The model under review builds one solid part; all positions refer to its coordinate system, in mm. A direction names the side the tool comes from. Coordinates: 2 decimals unless noted, no trailing zeros. Write each loop counter-clockwise with the first axis right and the second up, starting at its lowest first coordinate (ties: lowest second). Pieces come first, ordered by that corner, then holes. Notation, with made-up numbers: (47, 50.5) - (88, 50.5) arc R23 ccw to (88, 59.5) - close; hole circle Ø6 at (-22.75, 45). An arc over 180 degrees is marked (long way). Put each result on its own line as item: value.
from build123d import *

# Parameters (mm, degrees)
RESSALTO_EXTRUS_O1_DEPTH = 1.4
ESBO_O2_R                = 3.45
RESSALTO_EXTRUS_O2_DEPTH = 2.4
FURO4_D                  = 1.2
PADR_O_LINEAR1_COUNT     = 6
PADR_O_LINEAR1_PITCH     = 2
PADR_OCIRCULAR2_COUNT    = 2
PADR_OCIRCULAR2_COPY_1_D = 1.2
PADR_OCIRCULAR2_COPY_2_D = 1.2
PADR_OCIRCULAR2_COPY_3_D = 1.2
PADR_OCIRCULAR2_COPY_4_D = 1.2
PADR_OCIRCULAR2_COPY_5_D = 1.2
FURO1_D                  = 4.95
FURO1_DEPTH              = 2
FURO2_D                  = 4.6
FURO2_DEPTH              = 1
FURO3_D                  = 2.1


with BuildPart() as part:
    # Esboço1 → Ressalto-extrusão1 (new body)
    with BuildSketch(Plane(origin=(0, 0, 0), x_dir=(1, 0, 0), z_dir=(0, 1, 0))):
        with BuildLine():
            Line((-14.159121967, 1.99702088), (-2.209072203, 2.65))
            ThreePointArc((-2.209072203, 2.65), (3.45, 0), (-2.209072203, -2.65))
            Line((-2.209072203, -2.65), (-14.159121967, -1.99702088))
            ThreePointArc((-14.159121967, -1.99702088), (-16.05, 0), (-14.159121967, 1.99702088))
        make_face()
    ressalto_extrus_o1 = extrude(amount=-RESSALTO_EXTRUS_O1_DEPTH)

    # Esboço2 → Ressalto-extrusão2 (add)
    with BuildSketch(Plane.XZ.offset(1.4)):
        with Locations(Location((0, 0, 0), (0, 0, 90))):
            Circle(ESBO_O2_R)
    extrude(amount=RESSALTO_EXTRUS_O2_DEPTH)

    # Furo4 (through all)
    with Locations(Plane(origin=(0, 0, 0), x_dir=(1, 0, 0), z_dir=(0, 1, 0))):
        with Locations((-14.45, 0)):
            furo4 = Hole(FURO4_D / 2)

    # Padrão linear1: Furo4 ×6
    with Locations(*[(i * PADR_O_LINEAR1_PITCH, 0, 0) for i in range(1, PADR_O_LINEAR1_COUNT)]):
        add(furo4, mode=Mode.SUBTRACT)

    # PadrãoCircular2: Ressalto-extrusão1, Furo4 ×2 about axis
    padr_ocircular2_axis = Axis((0, 0, 0), (0, 1, 0))
    add([ressalto_extrus_o1.rotate(padr_ocircular2_axis, i * 360 / PADR_OCIRCULAR2_COUNT) for i in range(1, PADR_OCIRCULAR2_COUNT)])
    add([furo4.rotate(padr_ocircular2_axis, i * 360 / PADR_OCIRCULAR2_COUNT) for i in range(1, PADR_OCIRCULAR2_COUNT)], mode=Mode.SUBTRACT)

    # PadrãoCircular2 copy 1 (through all)
    with Locations(Plane(origin=(-2, 0, 0), x_dir=(-1, 0, 0), z_dir=(0, 1, 0))):
        with Locations((-14.45, 0)):
            Hole(PADR_OCIRCULAR2_COPY_1_D / 2)

    # PadrãoCircular2 copy 2 (through all)
    with Locations(Plane(origin=(-4, 0, 0), x_dir=(-1, 0, 0), z_dir=(0, 1, 0))):
        with Locations((-14.45, 0)):
            Hole(PADR_OCIRCULAR2_COPY_2_D / 2)

    # PadrãoCircular2 copy 3 (through all)
    with Locations(Plane(origin=(-6, 0, 0), x_dir=(-1, 0, 0), z_dir=(0, 1, 0))):
        with Locations((-14.45, 0)):
            Hole(PADR_OCIRCULAR2_COPY_3_D / 2)

    # PadrãoCircular2 copy 4 (through all)
    with Locations(Plane(origin=(-8, 0, 0), x_dir=(-1, 0, 0), z_dir=(0, 1, 0))):
        with Locations((-14.45, 0)):
            Hole(PADR_OCIRCULAR2_COPY_4_D / 2)

    # PadrãoCircular2 copy 5 (through all)
    with Locations(Plane(origin=(-10, 0, 0), x_dir=(-1, 0, 0), z_dir=(0, 1, 0))):
        with Locations((-14.45, 0)):
            Hole(PADR_OCIRCULAR2_COPY_5_D / 2)

    # Furo1
    with Locations(Plane(origin=(0, -3.8, 0), x_dir=(-1, 0, 0), z_dir=(0, -1, 0))):
        with Locations((0, 0)):
            Hole(FURO1_D / 2, depth=FURO1_DEPTH)

    # Furo2
    with Locations(Plane(origin=(0, 0, 0), x_dir=(1, 0, 0), z_dir=(0, 1, 0))):
        with Locations((0, 0)):
            Hole(FURO2_D / 2, depth=FURO2_DEPTH)

    # Furo3 (through all)
    with Locations(Plane(origin=(0, 0, 0), x_dir=(1, 0, 0), z_dir=(0, 1, 0))):
        with Locations((0, 0)):
            Hole(FURO3_D / 2)


solid = part.part
1. The part is to be moulded in two halves that separate along X. For faces 4 (the cylindrical face through (13.004, -0.71, -0.23)), 5 (the flat face through (0, 0, 3)), 6 (the flat face through (-8.1, -0.69, 2.33)), 7 (the cylindrical face through (15.004, -0.71, -0.23)), say which applies: +X half, -X half, draft (parallel to the pull), parting line (faces both ways), or undercut.
Determined:
face 4: undercut
face 5: draft
face 6: -X half
face 7: undercut
2. Machinability: for faces 1 (the cylindrical face through (16.05, -0.69, -0.04)), 2 (the cylindrical face through (2.36, -2.79, -0.74)), 3 (the flat face through (-1, -1, -1)), which of the approach directions +Z, -Z, +X, -X, +Y, -Y give a long, thin tool a straight path to every point of the face, cutting with its end or side? Answer none if there is none.
Determined:
face 1: +X, +Y, -Y
face 2: -Y
face 3: +Y
3. Consider section A-A on x = -6.45. State the section outline as (y, z) points, plus the area to 3 significant figures.
Determined:
outline: (-1.4, -2.42) - (0, -2.42) - (0, -0.6) - (-1.4, -0.6) - close; (-1.4, 0.6) - (0, 0.6) - (0, 2.42) - (-1.4, 2.42) - close
area: 5.09 mm^2
4. For pin 1 Ø1.6 at (x, z) = (9.5, 0) entering from -Y; pin 2 Ø3.5 at (x, z) = (-0.5, 0) entering from +Y, all flat-tipped, find the tip position at first contact; note any pin that passes through.
Determined:
pin 1: stops at y = -1.4
pin 2: stops at y = -1
5. To check wall thickness, follow probe 1 along Y at (x, z) = (12, 2); probe 2 along Z at (x, y) = (10.45, -0.6); probe 3 along Z at (x, y) = (14.5, -0.5). State the ranges of each line that lie inside material, in increasing order.
Determined:
probe 1: y = -1.4 to 0
probe 2: z = -2.2 to -0.6, 0.6 to 2.2
probe 3: z = -1.95 to -0.6, 0.6 to 1.95
6. Consider section B-B on y = -2.75. State the section outline as (x, z) points (3 decimals), plus the area to 3 significant figures.
Determined:
outline: circle Ø6.9 at (0, 0); hole circle Ø4.95 at (0, 0)
area: 18.1 mm^2
7. Consider section C-C on x = -1.5. State the section outline as (y, z) points.
Determined:
outline: (-3.8, -3.11) - (0, -3.11) - (0, -1.74) - (-1, -1.74) - (-1, 1.74) - (0, 1.74) - (0, 3.11) - (-3.8, 3.11) - (-3.8, 1.97) - (-1.8, 1.97) - (-1.8, -1.97) - (-3.8, -1.97) - close
8. Consider section D-D on x = -10.45. State the section outline as (y, z) points.
Determined:
outline: (-1.4, -2.2) - (0, -2.2) - (0, -0.6) - (-1.4, -0.6) - close; (-1.4, 0.6) - (0, 0.6) - (0, 2.2) - (-1.4, 2.2) - close
